Work out the finished part from the listing and answer in its coordinate system (mm). A direction names the side the tool comes from. Round coordinates to 2 decimals unless told otherwise and drop trailing zeros. Write each loop counter-clockwise with the first axis right and the second up, starting at its lowest first coordinate (ties: lowest second). Pieces come first, ordered by that corner, then holes. Notation, with made-up numbers: M -34.5,72.25 L -13.5,72.25 A8 cw -13.5,83.25 Z; hole C 36.5,77.5 d1. An arc over 180 degrees is marked long. One line per item, written item: value. Start each with the question number.
Q1. Find section A-A (z = 2.9). Write down the section's boundary in (x, y).
Q2. Find section D-D (z = 1.9). Write down the section's boundary in (x, y).
Q3. The mould has two halves that part along Y. Classify faces 5 (the cylindrical face through (6.449, -6.465, 1.972)), 6 (the flat face through (0, 5.75, 2)), 7 (the flat face through (6.75, 0, 1)): released by +Y, released by -Y, zero draft, split by the parting line, or undercut.
Q4. Given pin 1 Ø6 at (x, y) = (-2.5, -0.5) entering from -Z; pin 2 Ø1 at (x, z) = (-1.5, 2) entering from -Y; pin 3 Ø3 at (x, z) = (-1, 2) entering from -Y; pin 4 Ø5 at (x, y) = (5.5, -3.5) entering from -Z, each flat-ended and moving along its own axis, determine where each tip first touches the part or whether it passes through.
Q5. Find section B-B (y = -1.75). Write down the section's boundary in (x, z), and give its area (3 significant figures).
Q6. A tool of negligible diameter and unlimited length cuts with its end or side. For faces 1 (the cylindrical face through (6.465, 6.449, 1.972)), 2 (the cylindrical face through (-6.449, 6.465, 1.972)), 3 (the flat face through (5.75, 0, 2)), 4 (the flat face through (0, 0, 5)), from which of +Z, -Z, +X, -X, +Y, -Y can it reach the whole face along a straight path? Write none if from no direction.
Q7. Consider probe 1 along Y at (x, z) = (3.5, 2.95); probe 2 along X at (y, z) = (-0.5, 3.55). Determine where each line is inside the solid, lowest interval first.
from build123d import *

# Parameters (mm, degrees)
PAD_DEPTH          = 4
PAD001_DEPTH       = 1
FILLET_R           = 0.8
POLARPATTERN_COUNT = 4
POCKET_DEPTH       = 3.5


with BuildPart() as part:
    # Sketch → Pad (new body)
    with BuildSketch(Plane.XY):
        with BuildLine():
            Line((5.75, 6.75), (-5.75, 6.75))
            ThreePointArc((-5.75, 6.75), (-6.457107, 6.457107), (-6.75, 5.75))
            Line((-6.75, 5.75), (-6.75, -5.75))
            ThreePointArc((-6.75, -5.75), (-6.457107, -6.457107), (-5.75, -6.75))
            Line((-5.75, -6.75), (5.75, -6.75))
            ThreePointArc((5.75, -6.75), (6.457107, -6.457107), (6.75, -5.75))
            Line((6.75, -5.75), (6.75, 5.75))
            ThreePointArc((6.75, 5.75), (6.457107, 6.457107), (5.75, 6.75))
        make_face()
    extrude(amount=PAD_DEPTH)

    # Sketch001 (on Face10 of Pad) → Pad001 (join)
    with BuildSketch(Plane.XY.offset(4)):
        with BuildLine():
            Line((6.75, 8), (-6.75, 8))
            ThreePointArc((-6.75, 8), (-7.633883, 7.633883), (-8, 6.75))
            Line((-8, 6.75), (-8, -6.75))
            ThreePointArc((-8, -6.75), (-7.633883, -7.633883), (-6.75, -8))
            Line((-6.75, -8), (6.75, -8))
            ThreePointArc((6.75, -8), (7.633883, -7.633883), (8, -6.75))
            Line((8, -6.75), (8, 6.75))
            ThreePointArc((8, 6.75), (7.633883, 7.633883), (6.75, 8))
        make_face()
    extrude(amount=PAD001_DEPTH)

    # Fillet
    fillet_edges = [part.edges().sort_by_distance(p)[0] for p in [
        (0, -8, 5),
        (-7.633883, -7.633883, 5),
        (-8, 0, 5),
        (-7.633883, 7.633883, 5),
        (0, 8, 5),
        (7.633883, 7.633883, 5),
        (8, 0, 5),
        (7.633883, -7.633883, 5),
    ]]
    fillet(fillet_edges, radius=FILLET_R)

    # Sphere → Sphere (revolve)
    with BuildSketch(Plane(origin=(0, -6.75, 2), x_dir=(1, 0, 0), z_dir=(0, -1, 0))):
        with BuildLine():
            ThreePointArc((0, -0.5), (0.5, 0), (0, 0.5))
            Line((0, 0.5), (0, -0.5))
        make_face()
    sphere = revolve(axis=Axis((0, -6.75, 2), (0, 0, 1)))

    # PolarPattern: Sphere ×4 about axis
    polarpattern_axis = Axis((0, 0, 0), (0, 0, 1))
    for i in range(1, POLARPATTERN_COUNT):
        add(sphere.rotate(polarpattern_axis, i * 360 / POLARPATTERN_COUNT))

    # Sketch004 (on Face27 of PolarPattern) → Pocket (cut)
    with BuildSketch(Plane(origin=(0, -6.75, 0), x_dir=(1, 0, 0), z_dir=(0, 0, -1))):
        with BuildLine():
            Line((-5.75, -3), (-5.75, -10.5))
            ThreePointArc((-5.75, -10.5), (-5.164214, -11.914214), (-3.75, -12.5))
            Line((-3.75, -12.5), (3.75, -12.5))
            ThreePointArc((3.75, -12.5), (5.164214, -11.914214), (5.75, -10.5))
            Line((5.75, -10.5), (5.75, -3))
            ThreePointArc((5.75, -3), (5.164214, -1.585786), (3.75, -1))
            Line((3.75, -1), (-3.75, -1))
            ThreePointArc((-3.75, -1), (-5.164214, -1.585786), (-5.75, -3))
        make_face()
    extrude(amount=-POCKET_DEPTH, mode=Mode.SUBTRACT)


solid = part.part
The answers:
1. outline: M -6.75,-5.75 A1 ccw -5.75,-6.75 L 5.75,-6.75 A1 ccw 6.75,-5.75 L 6.75,5.75 A1 ccw 5.75,6.75 L -5.75,6.75 A1 ccw -6.75,5.75 Z; hole M -5.75,-3.75 A2 ccw -3.75,-5.75 L 3.75,-5.75 A2 ccw 5.75,-3.75 L 5.75,3.75 A2 ccw 3.75,5.75 L -3.75,5.75 A2 ccw -5.75,3.75 Z
2. outline: M -6.75,-5.75 A1 ccw -5.75,-6.75 L -0.49,-6.75 A0.49 ccw 0.49,-6.75 L 5.75,-6.75 A1 ccw 6.75,-5.75 L 6.75,-0.49 A0.49 ccw 6.75,0.49 L 6.75,5.75 A1 ccw 5.75,6.75 L 0.49,6.75 A0.49 ccw -0.49,6.75 L -5.75,6.75 A1 ccw -6.75,5.75 L -6.75,0.49 A0.49 ccw -6.75,-0.49 Z; hole M -5.75,-3.75 A2 ccw -3.75,-5.75 L 3.75,-5.75 A2 ccw 5.75,-3.75 L 5.75,3.75 A2 ccw 3.75,5.75 L -3.75,5.75 A2 ccw -5.75,3.75 Z
3. face 5: released by -Y
3. face 6: undercut
3. face 7: zero draft
4. pin 1: z = 3.5
4. pin 2: y = -6.75
4. pin 3: y = -7.25
4. pin 4: z = 0
5. outline: M -8,4 L -6.75,4 L -6.75,0 L -5.75,0 L -5.75,3.5 L 5.75,3.5 L 5.75,0 L 6.75,0 L 6.75,4 L 8,4 L 8,4.2 A0.8 ccw 7.2,5 L -7.2,5 A0.8 ccw -8,4.2 Z
5. area: 29.5 mm2
6. face 1: -Z, +X, +Y
6. face 2: -Z, -X, +Y
6. face 3: -Z
6. face 4: +Z, +X, -X, +Y, -Y
7. probe 1: -6.75 to -5.75, 5.75 to 6.75
7. probe 2: -6.75 to 6.75
